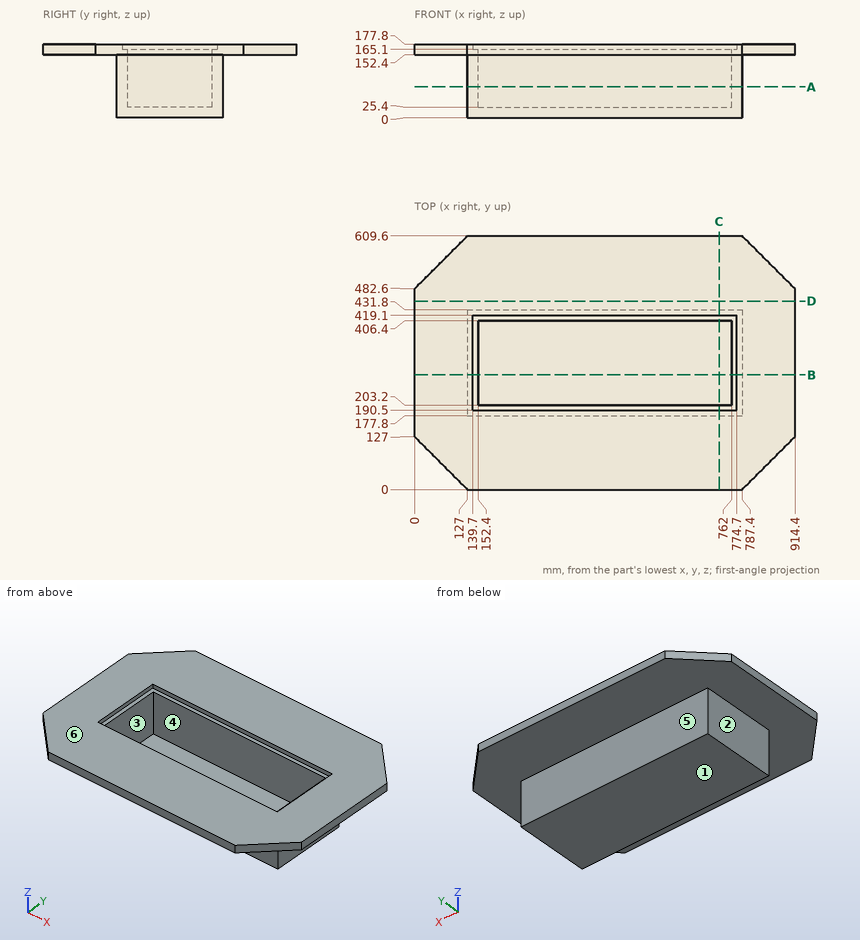
Source: three-view drawing plus pictorial views. Frame: mm from the lowest corner of the part. A direction names the side the tool comes from. Round coordinates to 2 decimals unless told otherwise and drop trailing zeros. Order: outer loops, then holes, each group sorted by start corner. A loop starts at its lowest first (then second) coordinate and runs counter-clockwise, first axis right, second up. Notation, with made-up numbers: (33, -30) - (74, -30) arc R15 cw to (74, -18) - close; hole circle Ø2 at (89, 45). An arc over 180 degrees is marked (long way). Answer in a Markdown table with one row per item.
Item 1: Section query B-B (y = 275.5). Return the cut outline in (x, z).
Model answer:
| item | result |
|---|---|
| outline | (0, 152.4) - (127, 152.4) - (127, 0) - (787.4, 0) - (787.4, 152.4) - (914.4, 152.4) - (914.4, 177.8) - (774.7, 177.8) - (774.7, 165.1) - (762, 165.1) - (762, 25.4) - (152.4, 25.4) - (152.4, 165.1) - (139.7, 165.1) - (139.7, 177.8) - (0, 177.8) - close |
Item 2: Section query C-C (x = 732). Return the cut outline in (y, z), then the cut area to 3 significant figures.
Model answer:
| item | result |
|---|---|
| outline | (0, 152.4) - (177.8, 152.4) - (177.8, 0) - (431.8, 0) - (431.8, 152.4) - (609.6, 152.4) - (609.6, 177.8) - (419.1, 177.8) - (419.1, 165.1) - (406.4, 165.1) - (406.4, 25.4) - (203.2, 25.4) - (203.2, 165.1) - (190.5, 165.1) - (190.5, 177.8) - (0, 177.8) - close |
| area | 22,900 mm² |
Item 3: Mould query, pull axis X, two halves, no side actions, for the marked faces 1, 2, 3 and 4. Classes: released by +X, released by -X, zero draft, split by the parting line, or undercut.
Model answer:
| item | result |
|---|---|
| face 1 | zero draft |
| face 2 | released by -X |
| face 3 | undercut |
| face 4 | undercut |
Item 4: Line query: line 1 (X direction, y = 325.5, z = 57); line 2 (X direction, y = 243, z = 160); line 3 (Y direction, x = 655, z = 102). Output: solid intervals per line, ascending.
Model answer:
| item | result |
|---|---|
| line 1 | x = 127 to 152.4, 762 to 787.4 |
| line 2 | x = 0 to 152.4, 762 to 914.4 |
| line 3 | y = 177.8 to 203.2, 406.4 to 431.8 |
Item 5: Section query D-D (y = 453). Return the cut outline in (x, z), then the cut area to 3 significant figures.
Model answer:
| item | result |
|---|---|
| outline | (0, 152.4) - (914.4, 152.4) - (914.4, 177.8) - (0, 177.8) - close |
| area | 23,200 mm² |
Item 6: Section query A-A (z = 75). Return the cut outline in (x, y), then the cut area to 3 significant figures.
Model answer:
| item | result |
|---|---|
| outline | (127, 177.8) - (787.4, 177.8) - (787.4, 431.8) - (127, 431.8) - close; hole (152.4, 203.2) - (762, 203.2) - (762, 406.4) - (152.4, 406.4) - close |
| area | 43,900 mm² |
Item 7: Pin query (flat end, axial travel): pin 1 (3 mm diameter, centred on y = 255, z = 80.5, fed in from -X); pin 2 (8 mm diameter, centred on x = 711, y = 281, fed in from +Z); pin 3 (8 mm diameter, centred on x = 137.5, z = 72.5, fed in from -Y); pin 4 (4 mm diameter, centred on x = 569.5, z = 172, fed in from -Y). Return the tip coordinate at first contact, or that it passes through.
Model answer:
| item | result |
|---|---|
| pin 1 | stops at x = 127 |
| pin 2 | stops at z = 25.4 |
| pin 3 | stops at y = 177.8 |
| pin 4 | stops at y = 0 |
Item 8: Reachability of the marked faces 5 and 6 from +Z, -Z, +X, -X, +Y, -Y: full face, straight path, thin tool, end or side. Return the list, or none.
Model answer:
| item | result |
|---|---|
| face 5 | -Z, +X, -X, +Y |
| face 6 | +Z, +X, -X, +Y, -Y |
